Input: part model. Units: mm. Frame: model coordinates. Round coordinates to 2 decimals unless told otherwise and drop trailing zeros. Loops run counter-clockwise (first coordinate to the right, second up) from the corner with the lowest first, then second, coordinate; pieces in that order, holes last. Notation, with made-up numbers: M 22,-16.75 L 40,-16.75 A9 ccw 40,-0.75 Z; hole C 17,-0.5 d5. An arc over 180 degrees is marked long. Return JSON: item names as keys, results as strings. Group by question number.
1) Section A-A (z = 2.05). Output: boundary loops of the cut face in (x, y).
2) Material intervals for line 1 (Y direction, x = 1.2, z = -0.5); line 2 (Y direction, x = 0.75, z = 2); line 3 (Z direction, x = 1.2, y = -21.5), sorted ascending. Write a range as from..to.
3) Section B-B (x = 1.35). Count the separate pieces of the cut face and the enclosed holes in it, plus the area to 3 significant figures.
4) Contact query for flat-ended pins moving along their axis: P1, Ø1.4, axis at x = 2, y = 23.5, coming from the +Z side; P2, Ø1, axis at y = 1, z = -4, coming from the -X side; P3, Ø1.4, axis at x = 1.5, y = -13, coming from the +Z side; P4, Ø1.1, axis at x = 1, z = 17.5, coming from the +Y side. Output: stop coordinate, or through.
5) Section C-C (z = -11.05). Output: boundary loops of the cut face in (x, y), plus the area to 3 significant figures.
from build123d import *

# Parameters (mm, degrees)
SKETCH_1_R          = 1.55
SKETCH_1_W          = 14
SKETCH_1_H          = 15
EXTRUDE_1_DEPTH     = 2.9
SKETCH_2_R          = 1.55
SKETCH_2_W          = 8
SKETCH_2_H          = 4.95
SKETCH_2_H_2        = 6
CUT_EXTRUDE_1_DEPTH = 10
FILLET_1_R          = 1


with BuildPart() as part:
    # 草图1 → 凸台-拉伸1 (new body)
    with BuildSketch(Plane(origin=(0, 0, 0), x_dir=(0, 0, -1), z_dir=(1, 0, 0))):
        with BuildLine():
            Line((-10.9, 25.45), (-10.9, 21.45))
            ThreePointArc((-10.9, 21.45), (-11.95, 20.4), (-13, 21.45))
            Line((-13, 21.45), (-18, 21.45))
            Line((-18, 21.45), (-18, 16.95))
            Line((-18, 16.95), (-18, 11.95))
            Line((-18, 11.95), (-18, -11.95))
            Line((-18, -11.95), (-18, -16.95))
            Line((-18, -16.95), (-18, -21.45))
            Line((-18, -21.45), (-13, -21.45))
            ThreePointArc((-13, -21.45), (-11.95, -20.4), (-10.9, -21.45))
            Line((-10.9, -21.45), (-10.9, -25.45))
            Line((-10.9, -25.45), (-3.1, -25.45))
            Line((-3.1, -25.45), (-3.1, -21.45))
            ThreePointArc((-3.1, -21.45), (-2.05, -20.4), (-1, -21.45))
            Line((-1, -21.45), (3, -21.45))
            ThreePointArc((3, -21.45), (4.05, -20.4), (5.1, -21.45))
            Line((5.1, -21.45), (5.1, -25.45))
            Line((5.1, -25.45), (12.9, -25.45))
            Line((12.9, -25.45), (12.9, -21.45))
            ThreePointArc((12.9, -21.45), (13.95, -20.4), (15, -21.45))
            Line((15, -21.45), (18, -21.45))
            Line((18, -21.45), (18, 21.45))
            Line((18, 21.45), (15, 21.45))
            ThreePointArc((15, 21.45), (13.95, 20.4), (12.9, 21.45))
            Line((12.9, 21.45), (12.9, 25.45))
            Line((12.9, 25.45), (5.1, 25.45))
            Line((5.1, 25.45), (5.1, 21.45))
            ThreePointArc((5.1, 21.45), (4.05, 20.4), (3, 21.45))
            Line((3, 21.45), (-1, 21.45))
            ThreePointArc((-1, 21.45), (-2.05, 20.4), (-3.1, 21.45))
            Line((-3.1, 21.45), (-3.1, 25.45))
            Line((-3.1, 25.45), (-10.9, 25.45))
        make_face()
        with Locations((-11, -8.95)):
            Circle(SKETCH_1_R, mode=Mode.SUBTRACT)
        with Locations((0, -8.95)):
            Rectangle(SKETCH_1_W, SKETCH_1_H, mode=Mode.SUBTRACT)
        with Locations((11, -8.95)):
            Circle(SKETCH_1_R, mode=Mode.SUBTRACT)
    extrude(amount=EXTRUDE_1_DEPTH)

    # 草图2 → 切除-拉伸1 (cut)
    with BuildSketch(Plane(origin=(2.9, 0, 0), x_dir=(0, 0, -1), z_dir=(1, 0, 0))):
        with Locations((10, 13.45)):
            Circle(SKETCH_2_R)
        with Locations((-10, 13.45)):
            Circle(SKETCH_2_R)
        with BuildLine():
            Line((-12.1, 3.425), (-12.1, 6.475))
            ThreePointArc((-12.1, 6.475), (-11.05, 7.525), (-10, 6.475))
            Line((-10, 6.475), (-6, 6.475))
            ThreePointArc((-6, 6.475), (-4.95, 7.525), (-3.9, 6.475))
            Line((-3.9, 6.475), (-3.9, 3.425))
            ThreePointArc((-3.9, 3.425), (-4.95, 2.375), (-6, 3.425))
            Line((-6, 3.425), (-10, 3.425))
            ThreePointArc((-10, 3.425), (-11.05, 2.375), (-12.1, 3.425))
        make_face()
        with BuildLine():
            Line((12.1, 3.4), (12.1, 6.5))
            ThreePointArc((12.1, 6.5), (11.05, 7.55), (10, 6.5))
            Line((10, 6.5), (6, 6.5))
            ThreePointArc((6, 6.5), (4.95, 7.55), (3.9, 6.5))
            Line((3.9, 6.5), (3.9, 3.4))
            ThreePointArc((3.9, 3.4), (4.95, 2.35), (6, 3.4))
            Line((6, 3.4), (10.002382304, 3.4))
            ThreePointArc((10.002382304, 3.4), (11.051191152, 2.4), (12.1, 3.4))
        make_face()
        with Locations((0, 13.975)):
            Rectangle(SKETCH_2_W, SKETCH_2_H)
        with Locations((-21, 8.5)):
            Rectangle(SKETCH_2_W, SKETCH_2_H_2)
        with Locations((-21, -13.5)):
            Rectangle(SKETCH_2_W, SKETCH_2_H_2)
    extrude(amount=-CUT_EXTRUDE_1_DEPTH, mode=Mode.SUBTRACT)

    # 圆角1
    fillet_1_edges = [part.edges().sort_by_distance(p)[0] for p in [
        (1.45, 16.45, -4),
        (1.45, 11.5, -4),
        (1.45, 11.5, 4),
        (1.45, 16.45, 4),
        (1.45, -16.45, 7),
        (1.45, -16.45, -7),
        (1.45, -1.45, -7),
        (1.45, -1.45, 7),
    ]]
    fillet(fillet_1_edges, radius=FILLET_1_R)


solid = part.part
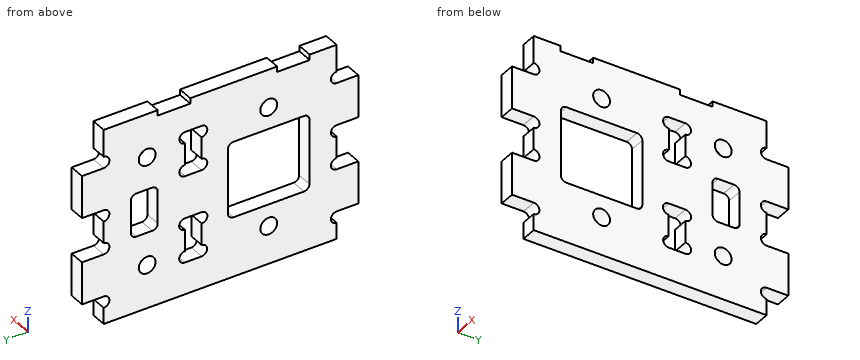
Returned:
{
 "1": {"outline": "M 0,-20.4 L 2.9,-20.4 L 2.9,-16.45 L 0,-16.45 Z; M 0,-1.45 L 2.9,-1.45 L 2.9,11.5 L 0,11.5 Z; M 0,16.45 L 2.9,16.45 L 2.9,20.4 L 0,20.4 Z"},
 "2": {"line 1": "y = -21.45..-16.45, -1.45..11.5, 16.45..21.45", "line 2": "y = -20.4..-16.45, -1.45..11.5, 16.45..20.4", "line 3": "z = -12.9..-5.1, 3.1..10.9"},
 "3": {"separate pieces": "1", "enclosed holes": "8", "area": "1,300 mm^2"},
 "4": {"P1": "stops at z = 10.9", "P2": "stops at x = 0", "P3": "stops at z = 17", "P4": "stops at y = 21.45"},
 "5": {"outline": "M 0,-25.45 L 2.9,-25.45 L 2.9,-10.5 L 0,-10.5 Z; M 0,-7.4 L 2.9,-7.4 L 2.9,2.4 L 0,2.4 Z; M 0,7.55 L 2.9,7.55 L 2.9,12.31 L 0,12.31 Z; M 0,14.59 L 2.9,14.59 L 2.9,25.45 L 0,25.45 Z", "area": "117 mm^2"}
}
